Verification items for the finished model (mm, model axes). Face numbers are marked on the shaded views. A direction names the side the tool comes from. Coordinates: 2 decimals unless noted, no trailing zeros. Write each loop counter-clockwise with the first axis right and the second up, starting at its lowest first coordinate (ties: lowest second). Pieces come first, ordered by that corner, then holes. Notation, with made-up numbers: M 67.5,82.5 L 92.5,82.5 A35 ccw 92.5,115.5 Z; hole C 1.25,-7 d6. An arc over 180 degrees is marked long. Answer in a Markdown table with one row per item.
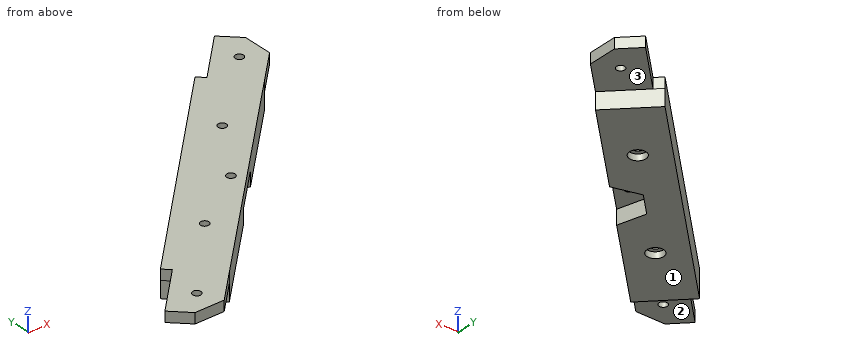
from build123d import *
from OCP.BRepFilletAPI import BRepFilletAPI_MakeChamfer

# Parameters (mm, degrees)
BOSS_EXTRUDE1_DEPTH = 5
SKETCH2_R           = 2
CUT_EXTRUDE1_DEPTH  = 15
BOSS_EXTRUDE2_DEPTH = 8
CHAMFER1_SIZE       = 10
CHAMFER1_SIZE2      = 9.982043079
CUT_EXTRUDE2_REACH  = 229.165
SKETCH4_R           = 2
SKETCH5_R           = 4
CUT_EXTRUDE3_DEPTH  = 3
CUT_EXTRUDE4_DEPTH  = 7
SKETCH7_R           = 2
CUT_EXTRUDE5_DEPTH  = 17


with BuildPart() as part:
    # Sketch1 → Boss-Extrude1 (new body)
    with BuildSketch(Plane.XY):
        Polygon((46.646446609, 27), (145, 125.000009716), (166.251364342, 146.174983473), (150.895154423, 161.531193392), (129.681985373, 140.318024342), (126.500004858, 143.500004858), (28.323223305, 45.323223305), (31.50520382, 42.141242789), (10.319228506, 20.955267476), (25.395082268, 5.825026243), align=None)
    extrude(amount=BOSS_EXTRUDE1_DEPTH)

    # Sketch2 → Cut-Extrude1 (cut)
    with BuildSketch(Plane.XY.offset(5)):
        with Locations((27.762116716, 23.256912896)):
            Circle(SKETCH2_R)
        with Locations((148.566315267, 144.061111447)):
            Circle(SKETCH2_R)
    extrude(amount=-CUT_EXTRUDE1_DEPTH, mode=Mode.SUBTRACT)

    # Sketch3 → Boss-Extrude2 (add)
    with BuildSketch(Plane(origin=(0, 0, 0), x_dir=(-1, 0, 0), z_dir=(0, 0, -1))):
        Polygon((-28.323223305, 45.323223305), (-46.613395502, 26.967067699), (-145, 125.000009716), (-126.500004858, 143.500004858), align=None)
    extrude(amount=BOSS_EXTRUDE2_DEPTH)

    # Chamfer1: one chamfer whose edges measure the first distance from different faces: ONE call of the kernel's chamfer builder (chamfer() names one face for all edges)
    chamfer1_edges_1 = [part.edges().sort_by_distance(p)[0] for p in [
        (25.395082268, 5.825026243, 2.5),
    ]]
    chamfer1_edges_2 = [part.edges().sort_by_distance(p)[0] for p in [
        (166.251364342, 146.174983473, 2.5),
    ]]
    chamfer1_side_2 = [part.faces().sort_by_distance(p)[0] for p in [
        (95.814501721, 75.991314625, -0.930462506),
    ]]
    chamfer1 = BRepFilletAPI_MakeChamfer(part.part.solid().wrapped)
    for e in chamfer1_edges_1:
        chamfer1.Add(CHAMFER1_SIZE, e.wrapped)
    for e in chamfer1_edges_2:
        chamfer1.Add(CHAMFER1_SIZE, CHAMFER1_SIZE2, e.wrapped, chamfer1_side_2[0].wrapped)  # the first distance lies on this face
    add(Compound.cast(chamfer1.Shape()), mode=Mode.REPLACE)

    # Sketch4 → Cut-Extrude2 (cut, up to next)
    with BuildSketch(Plane.XY.offset(5), mode=Mode.PRIVATE) as cut_extrude2_sk1:
        with Locations((62, 60)):
            Circle(SKETCH4_R)
    cut_extrude2_tool1 = extrude(cut_extrude2_sk1.sketch, amount=-CUT_EXTRUDE2_REACH, mode=Mode.PRIVATE) & part.part
    # Sketch4 → Cut-Extrude2 (cut, up to next)
    with BuildSketch(Plane.XY.offset(5), mode=Mode.PRIVATE) as cut_extrude2_sk2:
        with Locations((112, 110)):
            Circle(SKETCH4_R)
    cut_extrude2_tool2 = extrude(cut_extrude2_sk2.sketch, amount=-CUT_EXTRUDE2_REACH, mode=Mode.PRIVATE) & part.part
    add(cut_extrude2_tool1.solids().sort_by_distance((62, 60, 5))[0], mode=Mode.SUBTRACT)
    add(cut_extrude2_tool2.solids().sort_by_distance((112, 110, 5))[0], mode=Mode.SUBTRACT)

    # Sketch5 → Cut-Extrude3 (cut)
    with BuildSketch(Plane(origin=(0, 0, -8), x_dir=(-1, 0, 0), z_dir=(0, 0, -1))):
        with Locations(Location((-62, 60, 0), (0, 0, 90))):
            Circle(SKETCH5_R)
        with Locations(Location((-112, 110, 0), (0, 0, 90))):
            Circle(SKETCH5_R)
    extrude(amount=-CUT_EXTRUDE3_DEPTH, mode=Mode.SUBTRACT)

    # Sketch6 → Cut-Extrude4 (cut)
    with BuildSketch(Plane(origin=(0, 0, -8), x_dir=(-1, 0, 0), z_dir=(0, 0, -1))):
        Polygon((-92.220395862, 89.367799567), (-105.604656722, 85.781497678), (-109.190958611, 72.397236819), (-99.39299964, 62.599277847), (-86.00873878, 66.185579736), (-82.422436891, 79.569840596), align=None)
    extrude(amount=-CUT_EXTRUDE4_DEPTH, mode=Mode.SUBTRACT)

    # Sketch7 → Cut-Extrude5 (cut)
    with BuildSketch(Plane(origin=(0, 0, -1), x_dir=(-1, 0, 0), z_dir=(0, 0, -1))):
        with Locations(Location((-91.564057064, 80.226179394, 0), (0, 0, 90))):
            Circle(SKETCH7_R)
    extrude(amount=-CUT_EXTRUDE5_DEPTH, mode=Mode.SUBTRACT)


solid = part.part
1) Sectioned sample at B-B (y = 110). Record the cut outline in (x, z), then the cut area to 3 significant figures.
Response values:
| item | result |
|---|---|
| outline | M 93,-8 L 108,-8 L 108,-5 L 110,-5 L 110,5 L 93,5 Z; M 114,-5 L 116,-5 L 116,-8 L 129.95,-8 L 129.95,5 L 114,5 Z |
| area | 416 mm² |
2) Sectioned sample at D-D (y = 29.5). Record the cut outline in (x, z).
Response values:
| item | result |
|---|---|
| outline | M 18.86,0 L 44.09,0 L 44.09,-8 L 49.16,-8 L 49.16,5 L 18.86,5 Z |
3) Depth check by flat-ended pin: pin 1 (1.5 mm diameter, centred on y = 50.5, z = 2, fed in from +X); pin 2 (1 mm diameter, centred on y = 135, z = -4.5, fed in from -X); pin 3 (1 mm diameter, centred on x = 51, z = -4.5, fed in from -Y). Enter the tip coordinate at first touch or a pass-through.
Response values:
| item | result |
|---|---|
| pin 1 | stops at x = 70.98 |
| pin 2 | stops at x = 117.5 |
| pin 3 | stops at y = 30.84 |
4) Sectioned sample at A-A (x = 112). Record the cut outline in (y, z), then the cut area to 3 significant figures.
Response values:
| item | result |
|---|---|
| outline | M 92.12,-8 L 106,-8 L 106,-5 L 108,-5 L 108,5 L 92.12,5 Z; M 112,-5 L 114,-5 L 114,-8 L 129,-8 L 129,5 L 112,5 Z |
| area | 415 mm² |
5) Tool access check on the marked faces 1, 2 and 3. Record the directions out of +Z, -Z, +X, -X, +Y, -Y that give a thin tool (end or side, any length) a straight path to the whole face; none if there is none.
Response values:
| item | result |
|---|---|
| face 1 | -Z, +X, -X, +Y, -Y |
| face 2 | -Z, -X, -Y |
| face 3 | -Z, +X, +Y |
6) Sectioned sample at C-C (z = 2). Record the cut outline in (x, y), then the cut area to 3 significant figures.
Response values:
| item | result |
|---|---|
| outline | M 10.32,20.96 L 18.34,12.91 L 32.48,12.88 L 159.17,139.12 L 159.19,153.23 L 150.9,161.53 L 129.68,140.32 L 126.5,143.5 L 28.32,45.32 L 31.51,42.14 Z; hole C 27.76,23.26 d4; hole C 62,60 d4; hole C 91.56,80.23 d4; hole C 112,110 d4; hole C 148.57,144.06 d4 |
| area | 4,740 mm² |
7) Thickness scan on L1, parallel to Y at x = 111.5, z = -0.5; L2, parallel to X at y = 60, z = -7.15; L3, parallel to X at y = 108, z = -5.5. Record the ranges inside material, lowest first. Write a range as [from, to].
Response values:
| item | result |
|---|---|
| L1 | y = [91.62, 108.06], [111.94, 128.5] |
| L2 | x = [43, 58], [66, 79.77] |
| L3 | x = [91, 108.54], [115.46, 127.94] |
